Here's the drawing with two shaded views (mm, measured from the low corner). I have some questions. A direction names the side the tool comes from. Coordinates: 2 decimals unless noted, no trailing zeros. Write each loop counter-clockwise with the first axis right and the second up, starting at its lowest first coordinate (ties: lowest second). Pieces come first, ordered by that corner, then holes.
Item 1: We'd pull the mould along X, two halves only. Please class the marked faces 6, 7 and 8: +X half, -X half, draft (parallel to the pull), parting line (faces both ways), or undercut.
Item 2: For the marked faces 1, 2, 3, 4 and 5, which set-ups out of +Z, -Z, +X, -X, +Y, -Y let a thin tool reach every point of the face, with its end or its side?
Item 3: If we section it at C-C (x = 35): Please give me the cut outline in (y, z).
Item 4: If we section it at D-D (y = 4): Please give me the cut outline in (x, z).
Item 5: If we section it at A-A (x = 8.5): Please give me the cut outline in (y, z), then the cut area to 3 significant figures.
Item 6: I'm going to push flat-ended pins straight in: pin 1 Ø12.5 at (y, z) = (34, 48) entering from +X; pin 2 Ø2 at (x, z) = (40, 18.5) entering from +Y; pin 3 Ø9 at (x, y) = (37.5, 33) entering from +Z; pin 4 Ø1 at (x, z) = (47.5, 28.5) entering from -Y. Where does each tip first touch, or does it pass through?
Item 7: If we section it at B-B (z = 5): Please give me the cut outline in (x, y).
Item 8: If I drill on line 1 (X direction, y = 42.5, z = 41); line 2 (Y direction, x = 62, z = 50); line 3 (X direction, y = 30, z = 5.5), over which ranges is the centre line in solid material (lowest first)?
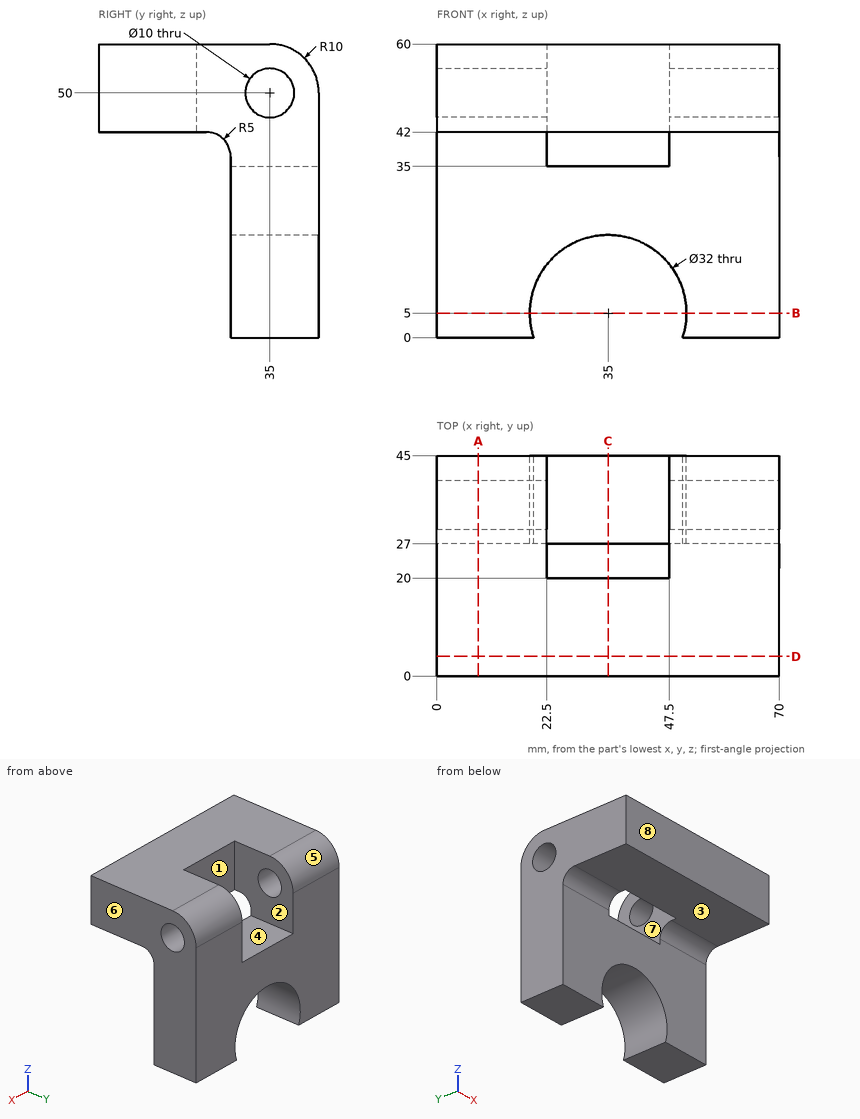
Answer list:
1. face 6: +X half
1. face 7: undercut
1. face 8: draft
2. face 1: +Z, -Z, +Y
2. face 2: +Z, +Y
2. face 3: -Z, +X, -X, -Y
2. face 4: +Z, +Y, -Y
2. face 5: +Z, +X, -X, +Y
3. outline: (0, 42) - (20, 42) - (20, 60) - (0, 60) - close; (27, 21) - (45, 21) - (45, 35) - (27, 35) - close
4. outline: (0, 42) - (70, 42) - (70, 60) - (0, 60) - close
5. outline: (0, 42) - (22, 42) arc R5 cw to (27, 37) - (27, 0) - (45, 0) - (45, 50) arc R10 ccw to (35, 60) - (0, 60) - close; hole circle Ø10 at (35, 50)
5. area: 1,470 mm2
6. pin 1: stops at x = 70
6. pin 2: passes through
6. pin 3: stops at z = 35
6. pin 4: stops at y = 27
7. outline: (0, 27) - (19, 27) - (19, 45) - (0, 45) - close; (51, 27) - (70, 27) - (70, 45) - (51, 45) - close
8. line 1: x = 0 to 22.5, 47.5 to 70
8. line 2: y = 0 to 30, 40 to 45
8. line 3: x = 0 to 19.01, 50.99 to 70
